Here's the drawing with two shaded views (mm, measured from the low corner). I have some questions. A direction names the side the tool comes from. Coordinates: 2 decimals unless noted, no trailing zeros. Loops run counter-clockwise (first coordinate to the right, second up) from the corner with the lowest first, then second, coordinate; pieces in that order, holes last. Notation, with made-up numbers: M 16.5,73 L 61.5,73 A27 ccw 61.5,108 Z; hole C 75.5,-2 d8. An arc over 180 degrees is marked long. Return JSON: item names as keys, results as strings. Group by question number.
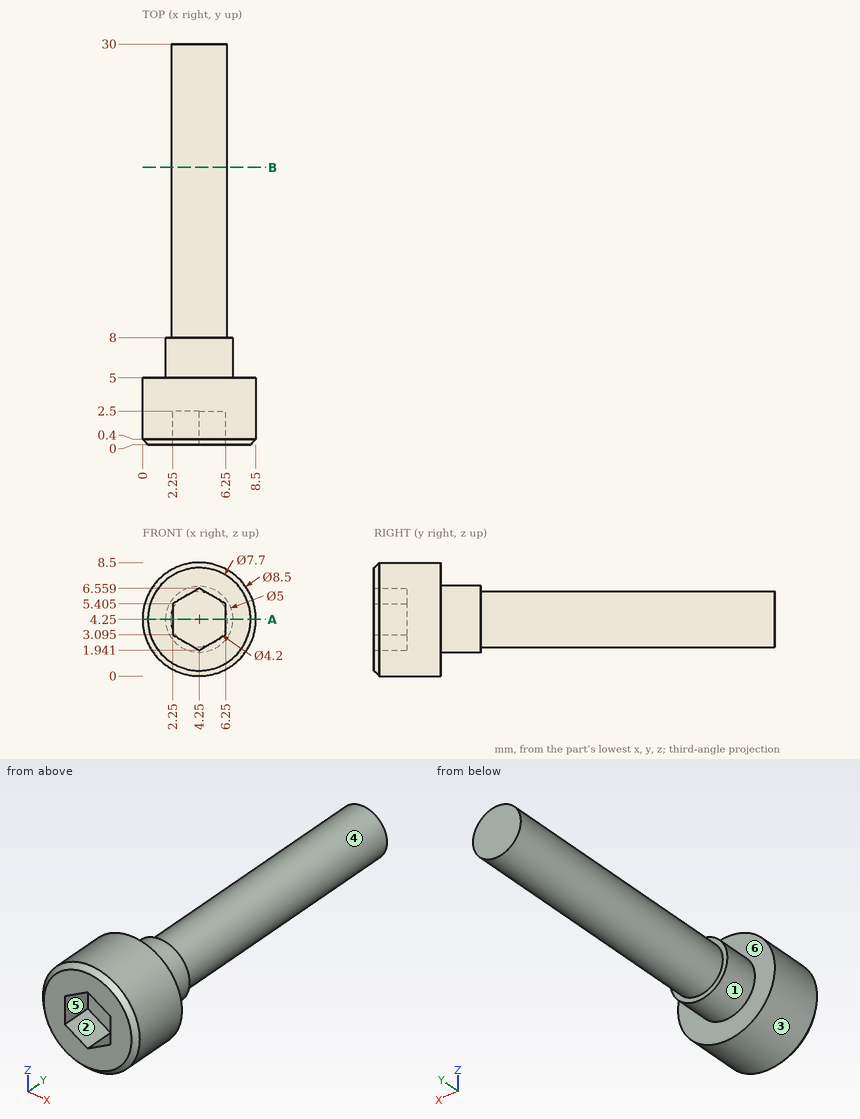
1) If we mould it in two halves opening along Z, with no side actions, what happens to the marked faces 4, 5 and 6? For each: +Z half, -Z half, draft (parallel to the pull), parting line (faces both ways), or undercut.
2) If I drill on line 1 (Y direction, x = 5.5, z = 2); line 2 (Z direction, x = 2.75, y = 7.75); line 3 (Y direction, x = 5.25, z = 2), over which ranges is the centre line in solid material (lowest first)? Write a range as from..to.
3) For pin 1 (3 mm diameter, centred on x = 2.5, y = 7.5, fed in from -Z); pin 2 (2 mm diameter, centred on x = 4.5, z = 3.5, fed in from -Y), each with a flat end and sliding along its axis, tell me the tip position at first contact or that it passes through.
4) For the marked faces 1, 2 and 3, which set-ups out of +Z, -Z, +X, -X, +Y, -Y let a thin tool reach every point of the face, with its end or its side?
5) Suppose I cut it at B-B, the plane y = 20.75. List the corners of the cut face in (x, z) for me.
6) Suppose I cut it at A-A, the plane z = 4.25. List the corners of the cut face in (x, y) for me.
Returned:
{
 "1": {"face 4": "parting line", "face 5": "undercut", "face 6": "draft"},
 "2": {"line 1": "y = 0..5", "line 2": "z = 2.25..6.25", "line 3": "y = 0..8"},
 "3": {"pin 1": "stops at z = 1.76", "pin 2": "stops at y = 2.5"},
 "4": {"face 1": "+Y", "face 2": "-Y", "face 3": "+Y, -Y"},
 "5": {"outline": "C 4.25,4.25 d4.2"},
 "6": {"outline": "M 0,0.4 L 0.4,0 L 2.25,0 L 2.25,2.5 L 6.25,2.5 L 6.25,0 L 8.1,0 L 8.5,0.4 L 8.5,5 L 6.75,5 L 6.75,8 L 6.35,8 L 6.35,30 L 2.15,30 L 2.15,8 L 1.75,8 L 1.75,5 L 0,5 Z"}
}
